```python
from build123d import *

# Parameters (mm, degrees)
BOSS_EXTRUDE1_DEPTH     = 20
SKETCH3_R               = 1.5
CUT_EXTRUDE1_DEPTH      = 1
CUT_EXTRUDE1_DEPTH_BACK = 2
SKETCH17_R              = 1.5
CUT_EXTRUDE13_DEPTH     = 2
SKETCH4_R               = 1.5
CUT_EXTRUDE2_DEPTH      = 1
CUT_EXTRUDE2_DEPTH_BACK = 18
BOSS_EXTRUDE2_DEPTH     = 111.6
SKETCH7_R               = 7.5
CUT_EXTRUDE3_DEPTH      = 18
LPATTERN1_COUNT         = 5
LPATTERN1_PITCH         = 19.15
SKETCH8_R               = 1.1
CUT_EXTRUDE4_DEPTH      = 18
CUT_EXTRUDE6_DEPTH      = 26
CUT_EXTRUDE7_DEPTH      = 26
CUT_EXTRUDE8_DEPTH      = 26
CUT_EXTRUDE9_DEPTH      = 26
CUT_EXTRUDE10_DEPTH     = 26
LPATTERN2_COUNT         = 3
LPATTERN2_PITCH         = 36.4853
LPATTERN3_COUNT         = 3
LPATTERN3_PITCH         = 36.4853
LPATTERN4_COUNT         = 2
LPATTERN4_PITCH         = 36.4853
LPATTERN5_COUNT         = 2
LPATTERN5_PITCH         = 36.4853
CUT_EXTRUDE11_DEPTH     = 26
SKETCH16_R              = 2.05
CUT_EXTRUDE12_DEPTH     = 18
SKETCH18_W              = 7
SKETCH18_H              = 3
CUT_EXTRUDE14_DEPTH     = 2
FILLET1_R               = 1


with BuildPart() as part:
    # Sketch1 → Boss-Extrude1 (new body)
    with BuildSketch(Plane.XY):
        with BuildLine():
            Line((-12.5, -8.5), (-10.5, -8.5))
            Line((-10.5, -8.5), (-10.5, 4.5))
            ThreePointArc((-10.5, 4.5), (-9.914213562, 5.914213562), (-8.5, 6.5))
            Line((-8.5, 6.5), (8.5, 6.5))
            ThreePointArc((8.5, 6.5), (9.914213562, 5.914213562), (10.5, 4.5))
            Line((10.5, 4.5), (10.5, -8.5))
            Line((10.5, -8.5), (12.5, -8.5))
            Line((12.5, -8.5), (12.5, 6.5))
            ThreePointArc((12.5, 6.5), (11.914213562, 7.914213562), (10.5, 8.5))
            Line((10.5, 8.5), (-10.5, 8.5))
            ThreePointArc((-10.5, 8.5), (-11.914213562, 7.914213562), (-12.5, 6.5))
            Line((-12.5, 6.5), (-12.5, -8.5))
        make_face()
    extrude(amount=BOSS_EXTRUDE1_DEPTH)

    # Sketch3 → Cut-Extrude1 (cut, two sides)
    with BuildSketch(Plane(origin=(12.5, 0, 0), x_dir=(0, 0, -1), z_dir=(1, 0, 0))) as cut_extrude1_sk:
        with Locations((-15, -1)):
            Circle(SKETCH3_R)
    extrude(amount=CUT_EXTRUDE1_DEPTH, mode=Mode.SUBTRACT)
    extrude(cut_extrude1_sk.sketch, amount=-CUT_EXTRUDE1_DEPTH_BACK, mode=Mode.SUBTRACT)

    # Sketch17 → Cut-Extrude13 (cut)
    with BuildSketch(Plane.ZY.offset(12.5)):
        with Locations((5, -1)):
            Circle(SKETCH17_R)
    extrude(amount=-CUT_EXTRUDE13_DEPTH, mode=Mode.SUBTRACT)

    # Sketch4 → Cut-Extrude2 (cut, two sides)
    with BuildSketch(Plane(origin=(0, 8.5, 0), x_dir=(1, 0, 0), z_dir=(0, 1, 0))) as cut_extrude2_sk:
        with Locations((-4.75, -15)):
            Circle(SKETCH4_R)
        with Locations((4.75, -5)):
            Circle(SKETCH4_R)
    extrude(amount=CUT_EXTRUDE2_DEPTH, mode=Mode.SUBTRACT)
    extrude(cut_extrude2_sk.sketch, amount=-CUT_EXTRUDE2_DEPTH_BACK, mode=Mode.SUBTRACT)

    # Sketch6 → Boss-Extrude2 (add)
    with BuildSketch(Plane.XY.offset(20)):
        with BuildLine():
            Line((-12.5, 6.5), (-12.5, -8.5))
            Line((-12.5, -8.5), (-10.5, -8.5))
            Line((-10.5, -8.5), (-10.5, 4.5))
            ThreePointArc((-10.5, 4.5), (-9.914213562, 5.914213562), (-8.5, 6.5))
            Line((-8.5, 6.5), (8.5, 6.5))
            ThreePointArc((8.5, 6.5), (9.914213562, 5.914213562), (10.5, 4.5))
            Line((10.5, 4.5), (10.5, -8.5))
            Line((10.5, -8.5), (12.5, -8.5))
            Line((12.5, -8.5), (12.5, 6.5))
            ThreePointArc((12.5, 6.5), (11.914213562, 7.914213562), (10.5, 8.5))
            Line((10.5, 8.5), (-10.5, 8.5))
            ThreePointArc((-10.5, 8.5), (-11.914213562, 7.914213562), (-12.5, 6.5))
        make_face()
    extrude(amount=BOSS_EXTRUDE2_DEPTH)

    # Sketch7 → Cut-Extrude3 (cut, through all)
    with BuildSketch(Plane(origin=(0, 8.5, 0), x_dir=(1, 0, 0), z_dir=(0, 1, 0))):
        with Locations((0, -104.1)):
            Circle(SKETCH7_R)
    cut_extrude3 = extrude(amount=-CUT_EXTRUDE3_DEPTH, mode=Mode.SUBTRACT)

    # LPattern1: Cut-Extrude3 ×5
    with Locations(*[(0, 0, -i * LPATTERN1_PITCH) for i in range(1, LPATTERN1_COUNT)]):
        add(cut_extrude3, mode=Mode.SUBTRACT)

    # Sketch8 → Cut-Extrude4 (cut, through all)
    with BuildSketch(Plane(origin=(0, 8.5, 0), x_dir=(1, 0, 0), z_dir=(0, 1, 0))):
        with Locations((4.242640687, -117.357359313)):
            Circle(SKETCH8_R)
        with Locations((4.242640687, -125.842640687)):
            Circle(SKETCH8_R)
        with Locations((-4.242640687, -125.842640687)):
            Circle(SKETCH8_R)
        with Locations((-4.242640687, -117.357359313)):
            Circle(SKETCH8_R)
    extrude(amount=-CUT_EXTRUDE4_DEPTH, mode=Mode.SUBTRACT)

    # Sketch9 → Cut-Extrude6 (cut, through all)
    with BuildSketch(Plane(origin=(12.5, 0, 0), x_dir=(0, 0, -1), z_dir=(1, 0, 0))):
        Polygon((-131.6, 6.5), (-111.6, -8.5), (-131.6, -8.5), align=None)
    extrude(amount=-CUT_EXTRUDE6_DEPTH, mode=Mode.SUBTRACT)

    # Sketch10 → Cut-Extrude7 (cut, through all)
    with BuildSketch(Plane(origin=(12.5, 0, 0), x_dir=(0, 0, -1), z_dir=(1, 0, 0))):
        Polygon((-31, 4.5), (-20, 4.5), (-20, -6.5), align=None)
    cut_extrude7 = extrude(amount=-CUT_EXTRUDE7_DEPTH, mode=Mode.SUBTRACT)

    # Sketch11 → Cut-Extrude8 (cut, through all)
    with BuildSketch(Plane(origin=(12.5, 0, 0), x_dir=(0, 0, -1), z_dir=(1, 0, 0))):
        Polygon((-35.242640687, 4.5), (-24.242640687, -6.5), (-35.242640687, -6.5), align=None)
    cut_extrude8 = extrude(amount=-CUT_EXTRUDE8_DEPTH, mode=Mode.SUBTRACT)

    # Sketch12 → Cut-Extrude9 (cut, through all)
    with BuildSketch(Plane(origin=(12.5, 0, 0), x_dir=(0, 0, -1), z_dir=(1, 0, 0))):
        Polygon((-38.242640687, 4.5), (-38.242640687, -6.5), (-49.242640687, -6.5), align=None)
    cut_extrude9 = extrude(amount=-CUT_EXTRUDE9_DEPTH, mode=Mode.SUBTRACT)

    # Sketch13 → Cut-Extrude10 (cut, through all)
    with BuildSketch(Plane(origin=(12.5, 0, 0), x_dir=(0, 0, -1), z_dir=(1, 0, 0))):
        Polygon((-53.485281374, -6.5), (-42.485281374, 4.5), (-53.485281374, 4.5), align=None)
    cut_extrude10 = extrude(amount=-CUT_EXTRUDE10_DEPTH, mode=Mode.SUBTRACT)

    # LPattern2: Cut-Extrude7 ×3
    with Locations(*[(0, 0, i * LPATTERN2_PITCH) for i in range(1, LPATTERN2_COUNT)]):
        add(cut_extrude7, mode=Mode.SUBTRACT)

    # LPattern3: Cut-Extrude8 ×3
    with Locations(*[(0, 0, i * LPATTERN3_PITCH) for i in range(1, LPATTERN3_COUNT)]):
        add(cut_extrude8, mode=Mode.SUBTRACT)

    # LPattern4: Cut-Extrude9 ×2
    with Locations(*[(0, 0, i * LPATTERN4_PITCH) for i in range(1, LPATTERN4_COUNT)]):
        add(cut_extrude9, mode=Mode.SUBTRACT)

    # LPattern5: Cut-Extrude10 ×2
    with Locations(*[(0, 0, i * LPATTERN5_PITCH) for i in range(1, LPATTERN5_COUNT)]):
        add(cut_extrude10, mode=Mode.SUBTRACT)

    # Sketch14 → Cut-Extrude11 (cut, through all)
    with BuildSketch(Plane(origin=(12.5, 0, 0), x_dir=(0, 0, -1), z_dir=(1, 0, 0))):
        Polygon((-111.6, -6), (-111.6, 4.5), (-125.6, 4.5), align=None)
    extrude(amount=-CUT_EXTRUDE11_DEPTH, mode=Mode.SUBTRACT)

    # Sketch16 → Cut-Extrude12 (cut, through all)
    with BuildSketch(Plane(origin=(0, 8.5, 0), x_dir=(1, 0, 0), z_dir=(0, 1, 0))):
        with Locations((0, -121.6)):
            Circle(SKETCH16_R)
    extrude(amount=-CUT_EXTRUDE12_DEPTH, mode=Mode.SUBTRACT)

    # Sketch18 → Cut-Extrude14 (cut)
    with BuildSketch(Plane(origin=(0, 8.5, 0), x_dir=(1, 0, 0), z_dir=(0, 1, 0))):
        with BuildLine():
            ThreePointArc((-3.5, -128.6), (0, -126.990227771), (3.5, -128.6))
            Line((3.5, -128.6), (-3.5, -128.6))
        make_face()
        with Locations((0, -130.1)):
            Rectangle(SKETCH18_W, SKETCH18_H)
    extrude(amount=-CUT_EXTRUDE14_DEPTH, mode=Mode.SUBTRACT)

    # Fillet1
    fillet1_edges = [part.edges().sort_by_distance(p)[0] for p in [
        (-3.5, 7.5, 131.6),
        (3.5, 7.5, 131.6),
        (3.5, 7.5, 128.6),
        (-3.5, 7.5, 128.6),
    ]]
    fillet(fillet1_edges, radius=FILLET1_R)


solid = part.part
```
Design review of the part built by this model. Coordinates are the model's own, in mm. A direction names the side the tool comes from. Round coordinates to 2 decimals unless told otherwise and drop trailing zeros. Write each loop counter-clockwise with the first axis right and the second up, starting at its lowest first coordinate (ties: lowest second). Pieces come first, ordered by that corner, then holes.
Item 1: For probe 1 along X at (y, z) = (1.5, 38); probe 2 along Y at (x, z) = (5, 95.5); probe 3 along Y at (x, z) = (-11, 49), list the stretches that pass through material, from the lowest coordinate up.
Item 2: We need section A-A on x = 0. Write out the cut boundary in (y, z), and give its area (3 significant figures).
Item 3: We need section B-B on z = 5. Write out the cut boundary in (x, y).
Item 4: For faces 1 (the cylindrical face through (-4.386, 7.514, 116.267)), 2 (the flat face through (11.514, -1.077, 61.908)), 3 (the flat face through (-10.5, -2, 64)), list the 3-axis set-ups (+Z, -Z, +X, -X, +Y, -Y) from which the entire face can be reached by the end or side of a thin tool; tool diameter is ignored.
Item 5: The part is to be moulded in two halves that separate along Z. For faces 4 (the flat face through (11.51, -1.08, 43.82)), 5 (the flat face through (-12.5, -1, 65)), 6 (the flat face through (-1, 7, 0)), say which applies: +Z half, -Z half, draft (parallel to the pull), parting line (faces both ways), or undercut.
Item 6: Clearance check with flat-ended pins moving along their axes: pin 1 Ø2 at (x, z) = (4.24, 125.84) entering from +Y; pin 2 Ø2 at (x, y) = (-11.5, -2.5) entering from +Z; pin 3 Ø13.5 at (x, z) = (2, 93) entering from -Y; pin 4 Ø2 at (x, y) = (-11.5, -1.5) entering from +Z. State where each tip first meets the part, or that it passes through.
Item 7: We need section C-C on z = 65.8. State how many separate pieces and enclosed holes the cut face has, and give its area (3 significant figures).
Returned:
1. probe 1: x = -12.5 to -10.5, 10.5 to 12.5
1. probe 2: y = 6.5 to 8.5
1. probe 3: y = -8.5 to -6.5, -6.26 to -2.01, 4.5 to 8.44
2. outline: (6.5, 0) - (8.5, 0) - (8.5, 20) - (6.5, 20) - close; (6.5, 35) - (8.5, 35) - (8.5, 39.15) - (6.5, 39.15) - close; (6.5, 54.15) - (8.5, 54.15) - (8.5, 58.3) - (6.5, 58.3) - close; (6.5, 73.3) - (8.5, 73.3) - (8.5, 77.45) - (6.5, 77.45) - close; (6.5, 92.45) - (8.5, 92.45) - (8.5, 96.6) - (6.5, 96.6) - close; (6.5, 111.6) - (8.5, 111.6) - (8.5, 119.55) - (6.5, 119.55) - close; (6.5, 123.65) - (8.5, 123.65) - (8.5, 126.99) - (6.5, 126.99) - close
2. area: 95.8 mm2
3. outline: (-12.5, -8.5) - (-10.5, -8.5) - (-10.5, -2.5) - (-12.5, -2.5) - close; (-12.5, 0.5) - (-10.5, 0.5) - (-10.5, 4.5) arc R2 cw to (-8.5, 6.5) - (3.25, 6.5) - (3.25, 8.5) - (-10.5, 8.5) arc R2 ccw to (-12.5, 6.5) - close; (6.25, 6.5) - (8.5, 6.5) arc R2 cw to (10.5, 4.5) - (10.5, -8.5) - (12.5, -8.5) - (12.5, 6.5) arc R2 ccw to (10.5, 8.5) - (6.25, 8.5) - close
4. face 1: +Y, -Y
4. face 2: +X, -X
4. face 3: +Z, -Z, -Y
5. face 4: undercut
5. face 5: draft
5. face 6: -Z half
6. pin 1: passes through
6. pin 2: stops at z = 120.93
6. pin 3: stops at y = 6.48
6. pin 4: stops at z = 122.27
7. separate pieces: 6
7. enclosed holes: 0
7. area: 53.0 mm2
